Answer from the drawing. Dimensions are ordinates in mm from the lowest x, y and z of the part. A direction names the side the tool comes from. Coordinates: 2 decimals unless noted, no trailing zeros. Write each loop counter-clockwise with the first axis right and the second up, starting at its lowest first coordinate (ties: lowest second). Pieces come first, ordered by that corner, then holes.
(1) The part is cut by section C-C, the plane x = 56. Determine the outline of the cut face in (y, z) (1 decimal).
(2) Given pin 1 (4 mm diameter, centred on y = 25.5, z = 17.5, fed in from +X); pin 2 (2 mm diameter, centred on x = 19, z = 26.5, fed in from -Y); pin 3 (12 mm diameter, centred on y = 22, z = 9, fed in from -X) (1 decimal), each flat-ended and moving along its own axis, determine where each tip first touches the part or whether it passes through.
(3) Which of the six approach directions +Z, -Z, +X, -X, +Y, -Y give full straight-line access (tool end or side, diameter ignored) to the marked faces 5 and 6?
(4) The part is cut by section D-D, the plane z = 22.5. Determine the outline of the cut face in (x, y) (1 decimal).
(5) Straight lines are drawn through the part: line 1 along Z through (x, y) = (13, 45); line 2 along Y through (x, z) = (56, 3.5) (1 decimal); line 3 along Y through (x, z) = (8.5, 17.5). For each, find the intervals that lie inside material, in ascending order.
(6) The part is cut by section A-A, the plane x = 37.5. Determine the outline of the cut face in (y, z) (1 decimal).
(7) Determine the mould class of the marked faces 1, 2, 3 and 4 for opening direction Z: pulls with the +Z half, pulls with the -Z half, needs draft (parallel to the pull), parting line crosses it, or undercut.
(8) The part is cut by section B-B, the plane y = 72. Determine the outline of the cut face in (x, z) (1 decimal).
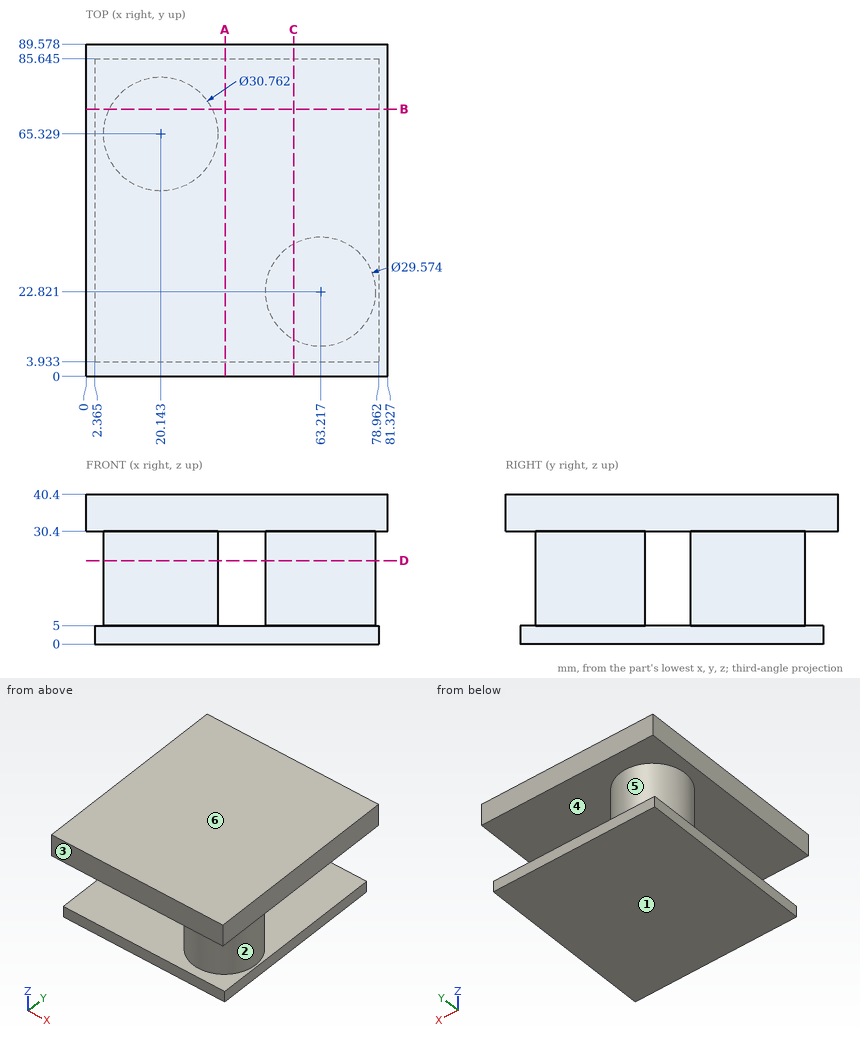
Computed:
1. outline: (0, 30.4) - (9.9, 30.4) - (9.9, 5) - (3.9, 5) - (3.9, 0) - (85.6, 0) - (85.6, 5) - (35.7, 5) - (35.7, 30.4) - (89.6, 30.4) - (89.6, 40.4) - (0, 40.4) - close
2. pin 1: stops at x = 77.99
2. pin 2: stops at y = 49.95
2. pin 3: stops at x = 2.4
3. face 5: none
3. face 6: +Z, +X, -X, +Y, -Y
4. outline: circle Ø30.8 at (20.1, 65.3); circle Ø29.6 at (63.2, 22.8)
5. line 1: z = 0 to 5, 30.4 to 40.4
5. line 2: y = 3.9 to 85.6
5. line 3: y = 55.28 to 75.38
6. outline: (0, 30.4) - (89.6, 30.4) - (89.6, 40.4) - (0, 40.4) - close; (3.9, 0) - (85.6, 0) - (85.6, 5) - (3.9, 5) - close
7. face 1: pulls with the -Z half
7. face 2: undercut
7. face 3: needs draft
7. face 4: undercut
8. outline: (0, 30.4) - (6.3, 30.4) - (6.3, 5) - (2.4, 5) - (2.4, 0) - (79, 0) - (79, 5) - (34, 5) - (34, 30.4) - (81.3, 30.4) - (81.3, 40.4) - (0, 40.4) - close
